For this review, take the finished solid that the model builds, in its own axes (mm). A direction names the side the tool comes from. Round coordinates to 2 decimals unless told otherwise and drop trailing zeros. Loops run counter-clockwise (first coordinate to the right, second up) from the corner with the lowest first, then second, coordinate; pieces in that order, holes last.
1) Take a section at C-C (z = 4.5). State the section outline as (x, y) points.
2) Wall thickness on L1, parallel to Y at x = -5.5, z = 4; L2, parallel to X at y = -5.5, z = 2; L3, parallel to Y at x = 20, z = 5.25: over which ranges is each line inside the solid? List them lowest first.
3) Take a section at B-B (y = 16). State the section outline as (x, z) points, then the cut area to 3 significant figures.
4) Take a section at A-A (x = 13.5). State the section outline as (y, z) points, then the cut area to 3 significant figures.
5) Mouldability with a two-part tool opening along X and no side actions: class faces 4 (the flat face through (24.25, 0, 4)), 5 (the flat face through (14, 21.25, 4)), 6 (the flat face through (-22.2, -22.3, 3.9)) as pulls with the +X half, pulls with the -X half, needs draft (parallel to the pull), parting line crosses it, or undercut.
6) Tool access review of faces 1 (the flat face through (12.5, 21.5, 0)), 2 (the flat face through (15.017, 32, 4)), 3 (the flat face through (0, 31.25, 4)): name each direction out of +Z, -Z, +X, -X, +Y, -Y from which nothing blocks a thin tool from reaching the whole face with its end or side.
7) Insertion check: pin 1 (2.5 mm diameter, centred on y = 35.5, z = 4.5, fed in from +X); pin 2 (1.6 mm diameter, centred on x = -16.5, z = 5.5, fed in from +Y); pin 3 (2.5 mm diameter, centred on y = 25, z = 3.5, fed in from +X). Each pin has a flat end and moves straight along its axis. Give the tip position at first contact, or say it passes through.
```python
from build123d import *

# Parameters (mm, degrees)
F1_DEPTH = 8
F2_SIZE  = 4
F3_W     = 11.25
F3_H     = 8
F4_DEPTH = 8


with BuildPart() as f1:
    # F0 (on Top) → F1 (new body)
    with BuildSketch(Plane.XY):
        Polygon((21.25, 21.25), (21.25, -21.25), (-21.25, -21.25), (-21.25, 21.25), (-11.25, 21.25), (-11.25, 24.250001), (-24.250001, 24.250001), (-24.250001, -24.250001), (24.250001, -24.250001), (24.250001, 24.250001), (11.25, 24.250001), (11.25, 21.25), align=None)
    extrude(amount=F1_DEPTH)

    # F2
    f2_edges = [f1.edges().sort_by_distance(p)[0] for p in [
        (-21.25, 21.25, 4),
        (-21.25, -21.25, 4),
        (21.25, -21.25, 4),
        (-24.250001, -24.250001, 4),
        (-24.250001, 24.250001, 4),
        (24.250001, 24.250001, 4),
        (21.25, 21.25, 4),
        (24.250001, -24.250001, 4),
    ]]
    chamfer(f2_edges, length=F2_SIZE)

    # F3 (on face) → F4 (join)
    with BuildSketch(Plane(origin=(0, 0, 0), x_dir=(1, 0, 0), z_dir=(0, 0, -1))):
        Polygon((-11.25, -31.250001), (-11.25, -24.250001), (-15.016655, -24.250001), (-15.016655, -39.250001), (-11.25, -39.250001), align=None)
        with Locations((-5.625, -35.250001)):
            Rectangle(F3_W, F3_H)
        with Locations((5.625, -35.250001)):
            Rectangle(F3_W, F3_H)
        Polygon((11.25, -24.250001), (11.25, -31.250001), (11.25, -39.250001), (15.016655, -39.250001), (15.016655, -24.250001), align=None)
    extrude(amount=-F4_DEPTH)


solid = f1.part
```
Response:
1. outline: (-24.25, -20.25) - (-20.25, -24.25) - (20.25, -24.25) - (24.25, -20.25) - (24.25, 20.25) - (20.25, 24.25) - (15.02, 24.25) - (15.02, 39.25) - (-15.02, 39.25) - (-15.02, 24.25) - (-20.25, 24.25) - (-24.25, 20.25) - close; hole (-21.25, -17.25) - (-17.25, -21.25) - (17.25, -21.25) - (21.25, -17.25) - (21.25, 17.25) - (17.25, 21.25) - (11.25, 21.25) - (11.25, 31.25) - (-11.25, 31.25) - (-11.25, 21.25) - (-17.25, 21.25) - (-21.25, 17.25) - close
2. L1: y = -24.25 to -21.25, 31.25 to 39.25
2. L2: x = -24.25 to -21.25, 21.25 to 24.25
2. L3: y = -24.25 to -18.5, 18.5 to 24.25
3. outline: (-24.25, 0) - (-21.25, 0) - (-21.25, 8) - (-24.25, 8) - close; (21.25, 0) - (24.25, 0) - (24.25, 8) - (21.25, 8) - close
3. area: 48.0 mm2
4. outline: (-24.25, 0) - (-21.25, 0) - (-21.25, 8) - (-24.25, 8) - close; (21.25, 0) - (39.25, 0) - (39.25, 8) - (21.25, 8) - close
4. area: 168 mm2
5. face 4: pulls with the +X half
5. face 5: undercut
5. face 6: pulls with the -X half
6. face 1: -Z, +X, -X, +Y, -Y
6. face 2: +Z, -Z, +X, +Y
6. face 3: +Z, -Z
7. pin 1: stops at x = 15.02
7. pin 2: stops at y = 24.25
7. pin 3: stops at x = 20.75
